For this review, take the finished solid that the model builds, in its own axes (mm). A direction names the side the tool comes from. Coordinates: 2 decimals unless noted, no trailing zeros. Write each loop counter-clockwise with the first axis right and the second up, starting at its lowest first coordinate (ties: lowest second). Pieces come first, ordered by that corner, then holes.
```python
from build123d import *

# Parameters (mm, degrees)
F1_DEPTH  = 90
F2_R      = 4.05
F3_DEPTH  = 25
F5_DEPTH  = 25
F6_R      = 1.75
F7_DEPTH  = 25
F9_R      = 3
F10_DEPTH = 25
F12_R     = 3
F13_DEPTH = 25
F14_SIZE  = 2
F15_R     = 1
F17_DEPTH = 1.5
F19_DEPTH = 1.5
F20_W     = 9.3469619751
F20_H     = 10.4837566614
F20_W_2   = 11.7468573153
F20_H_2   = 8.0838575959
F21_DEPTH = 90.001


with BuildPart() as f1:
    # F0 (on Top) → F1 (new body)
    with BuildSketch(Plane.XY):
        Polygon((70, 89), (61, 89), (11, 30), (11, 21), (19, 21), (19, 30), (19, 33.3303359461), (19, 37.1198922439), (56.1865319967, 81), (61, 81), (70, 81), align=None)
    extrude(amount=F1_DEPTH)

    # F2 (on face) → F3 (cut)
    with BuildSketch(Plane(origin=(-8.3947500418, 7.1141949507, 0), x_dir=(-0.6465216954, -0.7628956006, 0), z_dir=(-0.7628956006, 0.6465216954, 0))):
        with Locations((-88.5814800858, 27.5)):
            Circle(F2_R)
        with Locations((-88.5814800858, 62.5)):
            Circle(F2_R)
        with Locations((-68.6670692686, 45)):
            Circle(F2_R)
    extrude(amount=-F3_DEPTH, mode=Mode.SUBTRACT)

    # F4 (on face) → F5 (cut)
    with BuildSketch(Plane.XZ.offset(-21)):
        with BuildLine():
            ThreePointArc((16.75, 75), (16.2374368671, 76.2374368671), (15, 76.75))
            Line((15, 76.75), (15, 73.25))
            ThreePointArc((15, 73.25), (16.2374368671, 73.7625631329), (16.75, 75))
        make_face()
        with BuildLine():
            ThreePointArc((16.75, 15), (16.2374368671, 16.2374368671), (15, 16.75))
            Line((15, 16.75), (15, 13.25))
            ThreePointArc((15, 13.25), (16.2374368671, 13.7625631329), (16.75, 15))
        make_face()
        with BuildLine():
            Line((15, 13.25), (15, 16.75))
            ThreePointArc((15, 16.75), (13.25, 15), (15, 13.25))
        make_face()
        with BuildLine():
            Line((15, 73.25), (15, 76.75))
            ThreePointArc((15, 76.75), (13.25, 75), (15, 73.25))
        make_face()
    extrude(amount=-F5_DEPTH, mode=Mode.SUBTRACT)

    # F6 (on face) → F7 (cut)
    with BuildSketch(Plane.YZ.offset(70)):
        with Locations((85, 75)):
            Circle(F6_R)
        with Locations((85, 15)):
            Circle(F6_R)
    extrude(amount=-F7_DEPTH, mode=Mode.SUBTRACT)

    # F9 (on offset) → F10 (cut)
    with BuildSketch(Plane.YZ.offset(65)):
        with Locations((85, 75)):
            Circle(F9_R)
        with Locations((85, 15)):
            Circle(F9_R)
    extrude(amount=-F10_DEPTH, mode=Mode.SUBTRACT)

    # F12 (on offset) → F13 (cut)
    with BuildSketch(Plane.XZ.offset(-26)):
        with Locations((15, 75)):
            Circle(F12_R)
        with Locations((15, 15)):
            Circle(F12_R)
    extrude(amount=-F13_DEPTH, mode=Mode.SUBTRACT)

    # F14
    f14_edges = [f1.edges().sort_by_distance(p)[0] for p in [
        (70, 81, 45),
        (70, 89, 45),
        (19, 21, 45),
        (11, 21, 45),
    ]]
    chamfer(f14_edges, length=F14_SIZE)

    # F15
    f15_edges = [f1.edges().sort_by_distance(p)[0] for p in [
        (61, 89, 45),
        (11, 30, 45),
    ]]
    fillet(f15_edges, radius=F15_R)

    # F16 (on face) → F17 (join)
    with BuildSketch(Plane.XY.offset(90)):
        Polygon((19, 37.1198922439), (19, 30.0599461219), (61, 30.0599461219), (61, 81), (56.1865319967, 81), align=None)
    extrude(amount=-F17_DEPTH)

    # F18 (on face) → F19 (join)
    with BuildSketch(Plane.XY):
        Polygon((61, 30), (61, 81), (56.1865319967, 81), (19, 37.1198922439), (19, 30), align=None)
    extrude(amount=F19_DEPTH)

    # F20 (on face) → F21 (cut, through all)
    with BuildSketch(Plane.XY.offset(90)):
        with Locations((67.2643706203, 84.9928185344)):
            Rectangle(F20_W, F20_H)
        with Locations((15.4358148575, 23.9219143987)):
            Rectangle(F20_W_2, F20_H_2)
    extrude(amount=-F21_DEPTH, mode=Mode.SUBTRACT)


solid = f1.part
```
1) Consider section D-D (y = 85). Give the boundary of the cut face in (x, z), then the cut area to 3 significant figures.
2) Clearance check with flat-ended pins moving along their axes: P1, Ø7, axis at y = 85, z = 15, coming from the -X side; P2, Ø5, axis at x = 59, z = 61.5, coming from the -Y side; P3, Ø1.2, axis at y = 64, z = 89, coming from the +X side; P4, Ø3.5, axis at x = 15, z = 75, coming from the -Y side. State where each tip first meets the part, or that it passes through.
3) Consider section A-A (x = 15). Give the boundary of the cut face in (y, z).
4) Tool access review of faces 4 (the face through (44, 50, 1.5)), 5 (the face through (62.591, 85, 46)): name each direction out of +Z, -Z, +X, -X, +Y, -Y from which nothing blocks a thin tool from reaching the whole face with its end or side.
5) The part is to be moulded in two halves that separate along Y. For faces 1 (the face through (42, 52, 90)), 2 (the face through (33.201, 53.877, 44.391)), 3 (the face through (60, 82, 15)), say which applies: pulls with the +Y half, pulls with the -Y half, needs draft (parallel to the pull), parting line crosses it, or undercut.
6) For L1, parallel to Z at x = 58, y = 85; L2, parallel to Z at x = 59, y = 74; L3, parallel to Y at x = 18, z = 48.5, list the stretches that pass through material, from the lowest coordinate up.
7) Consider section B-B (z = 15). Give the boundary of the cut face in (x, y).
8) Consider section C-C (z = 30). Give the boundary of the cut face in (x, y), then the cut area to 3 significant figures.
Results:
1. outline: (57.61, 0) - (62.59, 0) - (62.59, 12) - (57.61, 12) - close; (57.61, 18) - (62.59, 18) - (62.59, 72) - (57.61, 72) - close; (57.61, 78) - (62.59, 78) - (62.59, 90) - (57.61, 90) - close
1. area: 388 mm2
2. P1: stops at x = 54.64
2. P2: stops at y = 81
2. P3: stops at x = 61
2. P4: passes through
3. outline: (27.96, 0) - (34.72, 0) - (34.72, 12) - (27.96, 12) - close; (27.96, 18) - (34.72, 18) - (34.72, 72) - (27.96, 72) - close; (27.96, 78) - (34.72, 78) - (34.72, 90) - (27.96, 90) - close
4. face 4: +X, -Y
4. face 5: +Z, -Z, +X, +Y, -Y
5. face 1: needs draft
5. face 2: pulls with the -Y half
5. face 3: undercut
6. L1: z = 0 to 12, 18 to 72, 78 to 90
6. L2: z = 0 to 1.5, 88.5 to 90
6. L3: y = 27.96 to 38.26
7. outline: (11, 27.96) - (12, 27.96) - (12, 31.18) - (11.24, 30.28) arc R1 ccw to (11, 29.63) - close; (18, 27.96) - (19, 27.96) - (19, 37.12) - (56.19, 81) - (62.59, 81) - (62.59, 82) - (55.07, 82) - (18, 38.26) - close; (60.15, 88) - (62.59, 88) - (62.59, 89) - (61.46, 89) arc R1 ccw to (60.7, 88.65) - close
8. outline: (11, 27.96) - (19, 27.96) - (19, 37.12) - (47.96, 71.29) - (46.82, 72.26) - (11.24, 30.28) arc R1 ccw to (11, 29.63) - close; (50.94, 77.12) - (52.08, 76.15) - (56.19, 81) - (62.59, 81) - (62.59, 89) - (61.46, 89) arc R1 ccw to (60.7, 88.65) - close
8. area: 168 mm2
